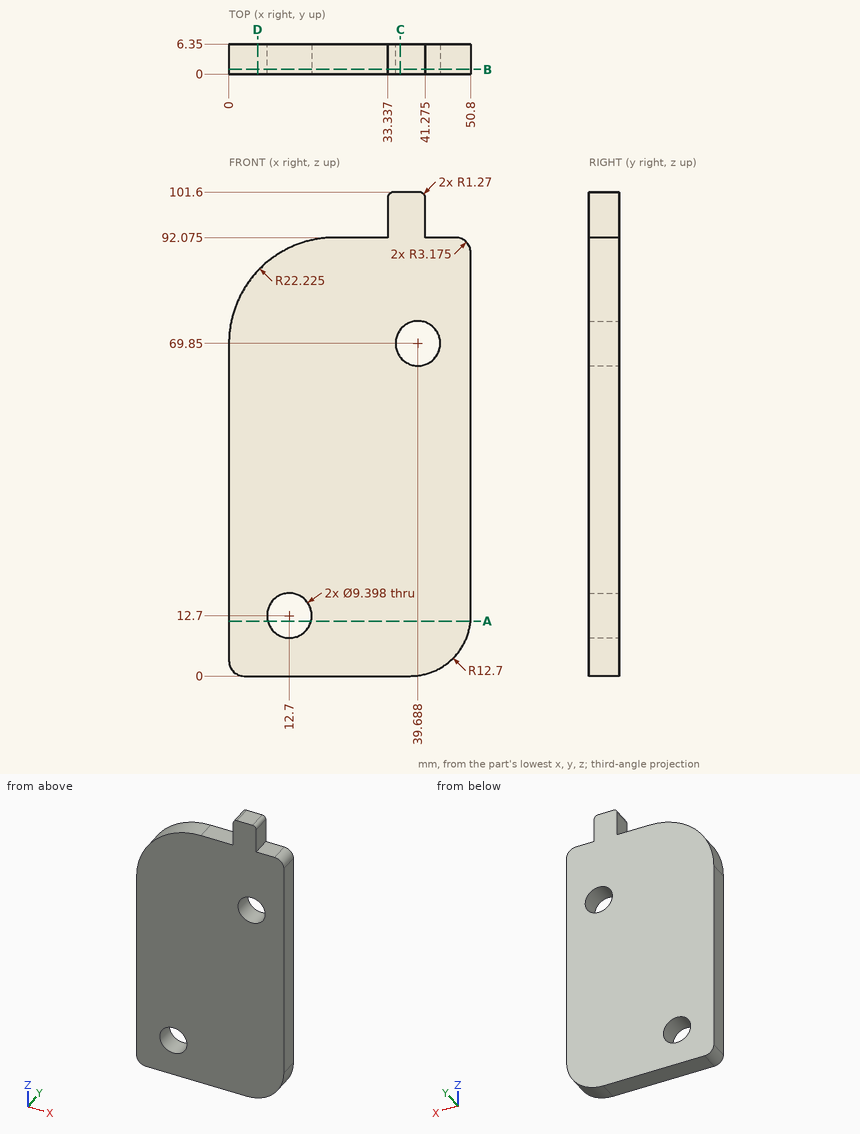
The drawing under review shows one solid part. Ordinate dimensions are in mm from its lowest x, y, z. Round coordinates to 2 decimals unless told otherwise and drop trailing zeros. Loops run counter-clockwise (first coordinate to the right, second up) from the corner with the lowest first, then second, coordinate; pieces in that order, holes last.
Item 1: For line 1 (X direction, y = 1, z = 13); line 2 (Z direction, x = 30, y = 2.25) (1 decimal); line 3 (Z direction, x = 40.5, y = 4.5), list the stretches that pass through material, from the lowest coordinate up.
Determined:
line 1: x = 0 to 8.01, 17.39 to 50.8
line 2: z = 0 to 92.1
line 3: z = 0.23 to 65.22, 74.48 to 101.5
Item 2: Take a section at A-A (z = 11.5). Write out the cut boundary in (x, y).
Determined:
outline: (0, 0) - (8.16, 0) - (8.16, 6.35) - (0, 6.35) - close; (17.24, 0) - (50.74, 0) - (50.74, 6.35) - (17.24, 6.35) - close
Item 3: Take a section at B-B (y = 1). Give the number of separate pieces and of enclosed holes in the cut face, then the cut area to 3 significant figures.
Determined:
separate pieces: 1
enclosed holes: 2
area: 4,470 mm2
Item 4: Clearance check with flat-ended pins moving along their axes: pin 1 Ø1.5 at (y, z) = (3, 71) entering from -X; pin 2 Ø7.5 at (x, z) = (39.69, 69.85) entering from +Y; pin 3 Ø1.9 at (x, y) = (45, 4) entering from +Z (1 decimal). State where each tip first meets the part, or that it passes through.
Determined:
pin 1: stops at x = 0
pin 2: passes through
pin 3: stops at z = 92.1
Item 5: Take a section at C-C (x = 36). Write out the cut boundary in (y, z), then the cut area to 3 significant figures.
Determined:
outline: (0, 0) - (6.35, 0) - (6.35, 66.94) - (0, 66.94) - close; (0, 72.76) - (6.35, 72.76) - (6.35, 101.6) - (0, 101.6) - close
area: 608 mm2
Item 6: Take a section at D-D (x = 6). Write out the cut boundary in (y, z), then the cut area to 3 significant figures.
Determined:
outline: (0, 0) - (6.35, 0) - (6.35, 85.04) - (0, 85.04) - close
area: 540 mm2
